Work out the finished part from the listing and answer in its coordinate system (mm). A direction names the side the tool comes from. Coordinates: 2 decimals unless noted, no trailing zeros. Loops run counter-clockwise (first coordinate to the right, second up) from the corner with the lowest first, then second, coordinate; pieces in that order, holes last. Notation, with made-up numbers: (-4, 36) -> (24, 36) arc R34 ccw to (24, 68) -> close; hole circle Ø6 at (71, 83.5). An arc over 180 degrees is marked (long way). Use a Markdown table: item, result.
Autodesk Fusion 360 part; units mm, degrees
sketch "Sketch1" plane through (0, 0, 0) normal (0, 1, 0) x (1, 0, 0)
  line L0 (20, -20) -> (-20, -20)
  line L1 (-20, -20) -> (-20, 20)
  line L2 (-20, 20) -> (20, 20)
  line L3 (20, 20) -> (20, -20)
  line L4 (20, -20) -> (-20, 20) construction
  line L5 (-20, -20) -> (20, 20) construction
  line L6 (-20, 4) -> (-15, 4)
  line L7 (-15, 4) -> (-15, -4)
  line L8 (-15, -4) -> (-20, -4)
  line L9 (-20, -4) -> (-20, 4)
  line L10 (-4, 20) -> (4, 20)
  line L11 (4, 20) -> (4, 15)
  line L12 (4, 15) -> (-4, 15)
  line L13 (-4, 15) -> (-4, 20)
  line L14 (20, 4) -> (15, 4)
  line L15 (15, 4) -> (15, -4)
  line L16 (15, -4) -> (20, -4)
  line L17 (20, -4) -> (20, 4)
  line L18 (-4, -20) -> (4, -20)
  line L19 (4, -20) -> (4, -15)
  line L20 (4, -15) -> (-4, -15)
  line L21 (-4, -15) -> (-4, -20)
  dimension "d1" = 40
  dimension "d2" = 40
  dimension "d3" = 5
  dimension "d4" = 8
  dimension "d5" = 16
  dimension "d6" = 5
  dimension "d7" = 16
  dimension "d8" = 8
  dimension "d9" = 5
  dimension "d10" = 5
  dimension "d11" = 8
  dimension "d12" = 8
  dimension "d13" = 16
  dimension "d14" = 16
extrude "Extrude1" add sketch "Sketch1" against normal blind 3 contours L0 L1 L2 L3 L6 L7 L8 L11 L12 L13 L14 L15 L16 L19 L20 L21
extrude "Extrude2" add sketch "Sketch1" against normal blind 8 contours L0 L18 L19 L20 L21 | L3 L14 L15 L16 L17 | L1 L6 L7 L8 L9 | L2 L10 L11 L12 L13
hole "Hole1" at (0, 0, 0) direction (0, -1, 0) diameter 9 depth 30 tip angle 118
fillet "Fillet1" radius 4 4 edges at (20, -1.5, -20) (-20, -1.5, -20) (20, -1.5, 20) (-20, -1.5, 20)
sketch "Sketch2" plane through (0, 0, 0) normal (0, 0, 1) x (1, 0, 0)
sketch "Sketch3" plane through (0, 0, 0) normal (0, 1, 0) x (1, 0, 0)
  line L0 (-10.5, 20) -> (10.5, 20)
  line L1 (10.5, 20) -> (10.5, 8)
  line L2 (10.5, 8) -> (-10.5, 8)
  line L3 (-10.5, 8) -> (-10.5, 20)
  line L4 (-20, -20) -> (-20, 20)
  dimension "d26" = 21
  dimension "d27" = 9.5
  dimension "d28" = 12
extrude "Extrude3" add sketch "Sketch3" along normal blind 80
sketch "Sketch4" plane through (0, 0, -8) normal (0, 0, 1) x (1, 0, 0)
  line L0 (-10.5, 0) -> (10.5, 0)
  line L1 (10.5, 0) -> (10.5, 80)
  line L2 (10.5, 80) -> (-10.5, 80)
  line L3 (-10.5, 80) -> (-10.5, 0)
  line L4 (-10.5, 80) -> (10.5, 80)
  line L5 (10.5, 80) -> (10.5, 59)
  line L6 (10.5, 59) -> (-10.5, 59)
  line L7 (-10.5, 59) -> (-10.5, 80)
  line L8 (8.5, 78) -> (8.5, 61)
  line L9 (8.5, 61) -> (-8.5, 61)
  line L10 (-8.5, 61) -> (-8.5, 78)
  line L11 (-8.5, 78) -> (8.5, 78)
  line L12 (-8.5, 78) -> (8.5, 78)
  line L13 (8.5, 78) -> (8.5, 67.7217)
  line L14 (8.5, 67.7217) -> (-8.5, 67.7217)
  line L15 (-8.5, 67.7217) -> (-8.5, 78)
  point P0 (-7.5, 64)
  point P1 (7.5, 64)
  dimension "d29" = 21
  dimension "d30" = 21
  dimension "d31" = 2
  dimension "d34" = 5
  dimension "d35" = 15
  dimension "d36" = 3
hole "Hole2" at (-7.5, 64, -8) at (7.5, 64, -8) direction (0, 0, -1) diameter 3 depth 55 tip angle 118
extrude "Extrude4" cut sketch "Sketch4" against normal blind 3 contours L8 L10 L11 L12 L13 L14 L15
sketch "Sketch5" plane through (0, 0, -20) normal (0, 0, -1) x (-1, 0, 0)
  circle A0 centre (7.5, 64) radius 1.5
  circle A1 centre (-7.5, 64) radius 1.5
  line L0 (16, -3) -> (16, 0)
  line L1 (16, 0) -> (10.5, 0)
  line L2 (10.5, 0) -> (10.5, 80)
  line L3 (10.5, 80) -> (-10.5, 80)
  line L4 (-10.5, 80) -> (-10.5, 0)
  line L5 (-10.5, 0) -> (-16, 0)
  line L6 (-16, 0) -> (-16, -3)
  line L7 (-16, -3) -> (-4, -3)
  line L8 (-4, -3) -> (-4, -8)
  line L9 (-4, -8) -> (4, -8)
  line L10 (4, -8) -> (4, -3)
  line L11 (4, -3) -> (16, -3)
  point P0 (-7.5, 64)
  point P1 (7.5, 64)
  point P2 (17, 58)
hole "Hole3" at (7.5, 64, -20) at (0, 0, 0) direction (0, 0, 1) diameter 5 depth 8 tip angle 118
equation "d6 = d3"
equation "d7 = d5"
equation "d8 = d4"
equation "d9 = d3"
equation "d10 = d3"
equation "d11 = d4"
equation "d12 = d4"
equation "d13 = d7"
equation "d14 = d7"
Q1. Consider line 1 (X direction, y = 64, z = -9); line 2 (X direction, y = 64, z = -15); line 3 (X direction, y = -0.8, z = 0). Determine where each line is inside the solid, lowest interval first. Write a range as [from, to].
Solved:
| item | result |
|---|---|
| line 1 | [-10.5, -9], [-6, 6], [9, 10.5] |
| line 2 | [-10.5, -9], [-6, 5], [10, 10.5] |
| line 3 | [-20, -4.5], [4.5, 20] |
Q2. Section C-C on z = 0 is taken. Determine the outline of the cut face in (x, y).
Solved:
| item | result |
|---|---|
| outline | (-20, -8) -> (-15, -8) -> (-15, -3) -> (-4.5, -3) -> (-4.5, 0) -> (-20, 0) -> close; (4.5, -3) -> (15, -3) -> (15, -8) -> (20, -8) -> (20, 0) -> (4.5, 0) -> close |
Q3. Determine the mould class of faces 4 (the flat face through (4, -5, -18)), 5 (the flat face through (8.5, 73, -9)), 6 (the cylindrical face through (-18.797, -1.521, 18.859)) for opening direction X: pulls with the +X half, pulls with the -X half, needs draft (parallel to the pull), parting line crosses it, or undercut.
Solved:
| item | result |
|---|---|
| face 4 | pulls with the +X half |
| face 5 | undercut |
| face 6 | pulls with the -X half |
Q4. Given pin 1 Ø5 at (x, z) = (-8, -5) entering from -Y; pin 2 Ø10 at (x, y) = (5, 58.5) entering from +Z; pin 3 Ø12 at (x, z) = (-6, -0.5) entering from +Y, each flat-ended and moving along its own axis, determine where each tip first touches the part or whether it passes through.
Solved:
| item | result |
|---|---|
| pin 1 | y = -3 |
| pin 2 | z = -8 |
| pin 3 | y = 0 |
Q5. For faces 1 (the flat face through (-17, -5, 4)), 2 (the flat face through (0, -5, -15)), 3 (the flat face through (0, 73, -11)), determine the directions among +Z, -Z, +X, -X, +Y, -Y from which every point of the face is accessible in a straight line to the end or side of a thin tool.
Solved:
| item | result |
|---|---|
| face 1 | +Z, +X, -X, -Y |
| face 2 | +X, -X, -Y |
| face 3 | +Z |
Q6. Section B-B on y = 64 is taken. Determine the outline of the cut face in (x, z), and give its area (3 significant figures).
Solved:
| item | result |
|---|---|
| outline | (-10.5, -20) -> (-9, -20) -> (-9, -8) -> (-10.5, -8) -> close; (-6, -20) -> (5, -20) -> (5, -12) -> (6, -11.4) -> (6, -8) -> (-6, -8) -> close; (9, -11.4) -> (10, -12) -> (10, -20) -> (10.5, -20) -> (10.5, -8) -> (9, -8) -> close |
| area | 163 mm² |
Q7. Section A-A on x = 0 is taken. Determine the outline of the cut face in (y, z), and give its area (3 significant figures).
Solved:
| item | result |
|---|---|
| outline | (-8, -20) -> (80, -20) -> (80, -8) -> (78, -8) -> (78, -11) -> (67.72, -11) -> (67.72, -8) -> (0, -8) -> (0, -4.5) -> (-3, -4.5) -> (-3, -15) -> (-8, -15) -> close; (-8, 15) -> (-3, 15) -> (-3, 4.5) -> (-2.5, 4.5) -> (-2.5, 8) -> (0, 9.5) -> (0, 20) -> (-8, 20) -> close |
| area | 1,060 mm² |
Q8. Section D-D on x = 7.5 is taken. Determine the outline of the cut face in (y, z).
Solved:
| item | result |
|---|---|
| outline | (-3, -20) -> (61.5, -20) -> (61.5, -12) -> (62.5, -11.4) -> (62.5, -8) -> (0, -8) -> (0, 20) -> (-3, 20) -> close; (65.5, -11.4) -> (66.5, -12) -> (66.5, -20) -> (80, -20) -> (80, -8) -> (78, -8) -> (78, -11) -> (67.72, -11) -> (67.72, -8) -> (65.5, -8) -> close |
